```python
from build123d import *

# Parameters (mm, degrees)
ESQUISSE1_R             = 1
ESQUISSE1_R_2           = 1.5
BOSS_EXTRU_1_DEPTH      = 5
ENL_V_MAT_EXTRU_1_DEPTH = 5
ESQUISSE3_W             = 20
ESQUISSE3_H             = 34
BOSS_EXTRU_2_DEPTH      = 5
ESQUISSE4_R             = 1.5
ESQUISSE4_W             = 9.798464728
ESQUISSE4_H             = 39.858161606
ENL_V_MAT_EXTRU_2_DEPTH = 5
ESQUISSE5_W             = 2.5
ESQUISSE5_H             = 34
BOSS_EXTRU_3_DEPTH      = 5
ESQUISSE6_R             = 1.6
BOSS_EXTRU_4_DEPTH      = 5
ESQUISSE7_W             = 28.704476199
ESQUISSE7_H             = 52.959758587
ENL_V_MAT_EXTRU_3_DEPTH = 10
ESQUISSE8_R             = 1
ESQUISSE8_R_2           = 1.5
BOSS_EXTRU_5_DEPTH      = 5
BOSS_EXTRU_6_DEPTH      = 49.5
BOSS_EXTRU_7_DEPTH      = 1
BOSS_EXTRU_7_DEPTH_BACK = 5


with BuildPart() as part:
    # Esquisse1 → Boss.-Extru.1 (new body)
    with BuildSketch(Plane.XY):
        with BuildLine():
            Line((-13.584596858, -30.047129187), (-13.584596858, -25.547129187))
            Line((-13.584596858, -25.547129187), (-13.584596858, -25.297129187))
            Line((-13.584596858, -25.297129187), (-13.834596858, -25.297129187))
            Line((-13.834596858, -25.297129187), (-16.334596858, -25.297129187))
            Line((-16.334596858, -25.297129187), (-16.584596858, -25.297129187))
            Line((-16.584596858, -25.297129187), (-16.584596858, -25.047129187))
            Line((-16.584596858, -25.047129187), (-16.584596858, 6.452870813))
            Line((-16.584596858, 6.452870813), (-16.584596858, 6.702870813))
            Line((-16.584596858, 6.702870813), (-16.334596858, 6.702870813))
            Line((-16.334596858, 6.702870813), (-13.834596858, 6.702870813))
            Line((-13.834596858, 6.702870813), (-13.584596858, 6.702870813))
            Line((-13.584596858, 6.702870813), (-13.584596858, 6.952870813))
            Line((-13.584596858, 6.952870813), (-13.584596858, 11.452870813))
            Line((-13.584596858, 11.452870813), (-13.584596858, 11.702870813))
            Line((-13.584596858, 11.702870813), (-13.334596858, 11.702870813))
            Line((-13.334596858, 11.702870813), (-8.584596858, 11.702870813))
            Line((-8.584596858, 11.702870813), (-8.584596858, 6.702870813))
            Line((-8.584596858, 6.702870813), (-7.491776281, 6.702870813))
            Line((-7.491776281, 6.702870813), (-4.034541178, 6.702870813))
            ThreePointArc((-4.034541178, 6.702870813), (-0.161557832, 6.19424756), (3.448773595, 4.702870813))
            ThreePointArc((3.448773595, 4.702870813), (10.66943645, 1.720117321), (18.415403142, 0.702870813))
            ThreePointArc((18.415403142, 0.702870813), (28.415403142, -9.297129187), (18.415403142, -19.297129187))
            ThreePointArc((18.415403142, -19.297129187), (10.66943645, -20.314375694), (3.448773595, -23.297129187))
            ThreePointArc((3.448773595, -23.297129187), (-0.161557832, -24.788505933), (-4.034541178, -25.297129187))
            Line((-4.034541178, -25.297129187), (-7.491776281, -25.297129187))
            Line((-7.491776281, -25.297129187), (-8.584596858, -25.297129187))
            Line((-8.584596858, -25.297129187), (-8.584596858, -30.297129187))
            Line((-8.584596858, -30.297129187), (-13.334596858, -30.297129187))
            Line((-13.334596858, -30.297129187), (-13.584596858, -30.297129187))
            Line((-13.584596858, -30.297129187), (-13.584596858, -30.047129187))
        make_face()
        with Locations((18.477857718, -2.297129187)):
            Circle(ESQUISSE1_R, mode=Mode.SUBTRACT)
        with Locations((25.415403142, -9.359583762)):
            Circle(ESQUISSE1_R, mode=Mode.SUBTRACT)
        with Locations((18.415403142, -9.297129187)):
            Circle(ESQUISSE1_R_2, mode=Mode.SUBTRACT)
        with Locations((11.415403142, -9.234674611)):
            Circle(ESQUISSE1_R, mode=Mode.SUBTRACT)
        with Locations((18.352948567, -16.297129187)):
            Circle(ESQUISSE1_R, mode=Mode.SUBTRACT)
    extrude(amount=BOSS_EXTRU_1_DEPTH)

    # Esquisse2 → Enlèv. mat.-Extru.1 (cut)
    with BuildSketch(Plane(origin=(0, 0, 0), x_dir=(-1, 0, 0), z_dir=(0, 0, -1))):
        Polygon((1.584596858, -19.297129187), (1.584596858, -25.297129187), (1.584596858, -26.297129187), (21.584596858, -26.297129187), (21.584596858, -33.65697819), (-26.833247513, -33.65697819), (-26.198667142, -19.297129187), align=None)
        Polygon((21.584596858, 7.702870813), (1.584596858, 7.702870813), (1.584596858, 6.702870813), (1.584596858, 0.702870813), (-26.198667142, 0.702870813), (-26.833247513, 15.062719816), (21.584596858, 15.062719816), align=None)
    extrude(amount=-ENL_V_MAT_EXTRU_1_DEPTH, mode=Mode.SUBTRACT)

    # Esquisse3 → Boss.-Extru.2 (add)
    with BuildSketch(Plane(origin=(0, 0, 0), x_dir=(-1, 0, 0), z_dir=(0, 0, -1))):
        with Locations((11.584596858, -9.297129187)):
            Rectangle(ESQUISSE3_W, ESQUISSE3_H)
    extrude(amount=-BOSS_EXTRU_2_DEPTH)

    # Esquisse4 → Enlèv. mat.-Extru.2 (cut)
    with BuildSketch(Plane(origin=(0, 0, 0), x_dir=(-1, 0, 0), z_dir=(0, 0, -1))):
        with Locations((9.084596858, -22.797129187)):
            Circle(ESQUISSE4_R)
        with Locations((9.084596858, 4.202870813)):
            Circle(ESQUISSE4_R)
        with Locations((23.983829222, -9.020336398)):
            Rectangle(ESQUISSE4_W, ESQUISSE4_H)
    extrude(amount=-ENL_V_MAT_EXTRU_2_DEPTH, mode=Mode.SUBTRACT)

    # Esquisse5 → Boss.-Extru.3 (add)
    with BuildSketch(Plane(origin=(0, 0, 0), x_dir=(-1, 0, 0), z_dir=(0, 0, -1))):
        with Locations((0.334596858, -9.297129187)):
            Rectangle(ESQUISSE5_W, ESQUISSE5_H)
    extrude(amount=-BOSS_EXTRU_3_DEPTH)

    # Esquisse6 → Boss.-Extru.4 (add)
    # profile 1 of 2: a face of its own
    with BuildSketch(Plane(origin=(0, 0, 0), x_dir=(-1, 0, 0), z_dir=(0, 0, -1))):
        with BuildLine():
            Line((12.324596858, -25.12480516), (5.844596858, -25.12480516))
            Line((5.844596858, -25.12480516), (5.844596858, -28.797129187))
            ThreePointArc((5.844596858, -28.797129187), (9.084596858, -32.037129187), (12.324596858, -28.797129187))
            Line((12.324596858, -28.797129187), (12.324596858, -25.12480516))
        make_face()
        with Locations((9.084596858, -28.797129187)):
            Circle(ESQUISSE6_R, mode=Mode.SUBTRACT)
    # profile 2 of 2: a face of its own
    with BuildSketch(Plane(origin=(0, 0, 0), x_dir=(-1, 0, 0), z_dir=(0, 0, -1))):
        with BuildLine():
            Line((12.324596858, 6.757738308), (5.844596858, 6.757738308))
            Line((5.844596858, 6.757738308), (5.844596858, 10.202870813))
            ThreePointArc((5.844596858, 10.202870813), (9.084596858, 13.442870813), (12.324596858, 10.202870813))
            Line((12.324596858, 10.202870813), (12.324596858, 6.757738308))
        make_face()
        with Locations((9.084596858, 10.202870813)):
            Circle(ESQUISSE6_R, mode=Mode.SUBTRACT)
    extrude(amount=-BOSS_EXTRU_4_DEPTH)

    # Esquisse7 → Enlèv. mat.-Extru.3 (cut)
    with BuildSketch(Plane.XY.offset(5)):
        with Locations((-12.936834958, -9.72769633)):
            Rectangle(ESQUISSE7_W, ESQUISSE7_H)
    extrude(amount=-ENL_V_MAT_EXTRU_3_DEPTH, mode=Mode.SUBTRACT)



with BuildPart() as body_2:
    # Esquisse8 → Boss.-Extru.5 (new body)
    with BuildSketch(Plane(origin=(0, 0, -39.5), x_dir=(-1, 0, 0), z_dir=(0, 0, -1))):
        with BuildLine():
            Line((-18.415403142, -19.297129187), (-1.415403142, -19.297129187))
            Line((-1.415403142, -19.297129187), (-1.415403142, 0.702870813))
            Line((-1.415403142, 0.702870813), (-18.415403142, 0.702870813))
            ThreePointArc((-18.415403142, 0.702870813), (-28.415403142, -9.297129187), (-18.415403142, -19.297129187))
        make_face()
        with Locations(Location((-11.415403142, -9.234674611, 0), (0, 0, 180))):
            Circle(ESQUISSE8_R, mode=Mode.SUBTRACT)
        with Locations(Location((-18.352948567, -16.297129187, 0), (0, 0, 180))):
            Circle(ESQUISSE8_R, mode=Mode.SUBTRACT)
        with Locations(Location((-18.415403142, -9.297129187, 0), (0, 0, 180))):
            Circle(ESQUISSE8_R_2, mode=Mode.SUBTRACT)
        with Locations(Location((-18.477857718, -2.297129187, 0), (0, 0, 180))):
            Circle(ESQUISSE8_R, mode=Mode.SUBTRACT)
        with Locations(Location((-25.415403142, -9.359583762, 0), (0, 0, 180))):
            Circle(ESQUISSE8_R, mode=Mode.SUBTRACT)
    extrude(amount=BOSS_EXTRU_5_DEPTH)


with BuildPart() as part_1:
    add(part.part)

    add(body_2.part)  # Boss.-Extru.6 merges body 2
    # Esquisse9 → Boss.-Extru.6 (add)
    with BuildSketch(Plane.XY.offset(5)):
        with BuildLine():
            Line((4.667676058, -19.297129187), (-1.1805148, -19.297129187))
            ThreePointArc((-1.1805148, -19.297129187), (-3.584596858, -9.297129187), (-1.1805148, 0.702870813))
            Line((-1.1805148, 0.702870813), (4.667676058, 0.702870813))
            ThreePointArc((4.667676058, 0.702870813), (1.415403142, -9.297129187), (4.667676058, -19.297129187))
        make_face()
    extrude(amount=-BOSS_EXTRU_6_DEPTH)

    # Esquisse10 → Boss.-Extru.7 (add, two sides: drawn at the far end of the back side and taken through both)
    with BuildSketch(Plane(origin=(-3.584596858, 0, 0), x_dir=(0, 0, -1), z_dir=(1, 0, 0)).offset(-BOSS_EXTRU_7_DEPTH_BACK)):
        Polygon((24.75, -12.183880533), (24.75, -6.410377841), (19.75, -3.523626495), (14.75, -6.410377841), (14.75, -12.183880533), (19.75, -15.070631878), align=None)
    extrude(amount=BOSS_EXTRU_7_DEPTH + BOSS_EXTRU_7_DEPTH_BACK)


solid = part_1.part
```
The listing builds one solid part. Answer for the finished solid, in the listing's coordinates (mm). A direction names the side the tool comes from. Coordinates: 2 decimals unless noted, no trailing zeros. Loops run counter-clockwise (first coordinate to the right, second up) from the corner with the lowest first, then second, coordinate; pieces in that order, holes last. Notation, with made-up numbers: M 58.5,-3.75 L 95.5,-3.75 A17 ccw 95.5,21.25 Z; hole C -39.75,-17.5 d9. An arc over 180 degrees is marked long. Answer as CSV lines item,"result". Start each with the question number.
(1) Given pin 1 (3 mm diameter, centred on x = 18.48, y = -2.3, fed in from +Z); pin 2 (4 mm diameter, centred on y = -7.5, z = -10.5, fed in from -X); pin 3 (2.5 mm diameter, centred on x = -5.5, y = -10, fed in from -Z); pin 4 (4 mm diameter, centred on x = -3.5, z = -38, fed in from +Y), each flat-ended and moving along its own axis, determine where each tip first touches the part or whether it passes through.
(2) The part is cut by section B-B (z = 1.5). Give the vertices of the cut face in (x, y), and give its area (3 significant figures).
(3) The part is cut by section D-D (z = -18). Give the vertices of the cut face in (x, y).
(4) For faces 1 (the flat face through (-5.739, -13.647, -22.215)), 2 (the flat face through (4, 0.703, -19)), 3 (the flat face through (-5.7, -13.6, -17.2)), determine the directions among +Z, -Z, +X, -X, +Y, -Y from which every point of the face is accessible in a straight line to the end or side of a thin tool.
(5) The part is cut by section A-A (x = 9). Give the vertices of the cut face in (y, z), and give its area (3 significant figures).
(6) The mould has two halves that part along Y. Classify faces 4 (the cylindrical face through (19.4, -1.91, -41.96)), 5 (the cylindrical face through (-3.584, -9.442, -13.904)), 6 (the flat face through (-5.74, -4.95, -17.28)), 7 (the cylindrical face through (19.277, -15.914, -41.965)): pulls with the +Y half, pulls with the -Y half, needs draft (parallel to the pull), parting line crosses it, or undercut.
(7) The part is cut by section C-C (y = -18). Give the vertices of the cut face in (x, z), and give its area (3 significant figures).
(8) Find the intervals of material crossed by L1, parallel to Z at x = 3, y = -3.5; L2, parallel to X at y = -8.5, z = 2; L3, parallel to Z at x = -4.5, y = -7, in increasing order. Write a range as [from, to].
Determined:
1,pin 1,"z = 5"
1,pin 2,"x = -3.58"
1,pin 3,"z = -24.75"
1,pin 4,"y = 0.05"
2,outline,"M -1.18,-19.3 L 18.42,-19.3 A10 ccw 18.42,0.7 L -1.18,0.7 A22 ccw Z; hole C 11.42,-9.23 d2; hole C 18.42,-9.3 d3; hole C 18.35,-16.3 d2; hole C 18.48,-2.3 d2; hole C 25.42,-9.36 d2"
2,area,"562 mm2"
3,outline,"M -8.58,-14.06 L -3.06,-14.06 A22 ccw -1.18,-19.3 L 4.67,-19.3 A17 cw 4.67,0.7 L -1.18,0.7 A22 ccw -3.06,-4.53 L -8.58,-4.53 Z"
4,face 1,"-Z, -X, -Y"
4,face 2,"+Z, -Z, +X, -X, +Y"
4,face 3,"+Z, -X, -Y"
5,outline,"M -19.3,-44.5 L 0.7,-44.5 L 0.7,-39.5 L -19.3,-39.5 Z; M -19.3,0 L 0.7,0 L 0.7,5 L -19.3,5 Z"
5,area,"200 mm2"
6,face 4,"undercut"
6,face 5,"parting line crosses it"
6,face 6,"pulls with the +Y half"
6,face 7,"undercut"
7,outline,"M -1.79,-44.5 L 23.34,-44.5 L 23.34,-39.5 L 3.81,-39.5 L 3.81,0 L 23.34,0 L 23.34,5 L -1.79,5 Z"
7,area,"473 mm2"
8,L1,"[-44.5, -39.5], [0, 5]"
8,L2,"[-3.57, 10.74], [12.09, 17.14], [19.69, 24.9], [25.93, 28.38]"
8,L3,"[-24.75, -14.75]"
